Source: CAD feature listing. Evaluate the final solid. Frame: model axes, mm. A direction names the side the tool comes from. Round coordinates to 2 decimals unless told otherwise and drop trailing zeros. Write each loop counter-clockwise with the first axis right and the second up, starting at its lowest first coordinate (ties: lowest second). Pieces come first, ordered by that corner, then holes. Notation, with made-up numbers: M -37,69 L 3,69 A29 cw 3,107 Z; hole C -39,-2 d10. An arc over 180 degrees is marked long. Use a Markdown table: item, result.
```python
from build123d import *

# Parameters (mm, degrees)
SKETCH1_W             = 128
SKETCH1_H             = 2.5
BOSS_EXTRUDE1_DEPTH   = 8
BOSS_EXTRUDE1_2_DEPTH = 8
SKETCH2_W             = 128
SKETCH2_H             = 21
BOSS_EXTRUDE2_DEPTH   = 3
SKETCH3_W             = 21
SKETCH3_H             = 17
BOSS_EXTRUDE3_DEPTH   = 2.5
SKETCH4_W             = 15
SKETCH4_H             = 21
BOSS_EXTRUDE4_DEPTH   = 2.5
SKETCH5_W             = 21
SKETCH5_H             = 39.5
BOSS_EXTRUDE5_DEPTH   = 2.5
FILLET1_R             = 5
SKETCH6_W             = 16
SKETCH6_H             = 8
CUT_EXTRUDE1_DEPTH    = 18.5
FILLET2_R             = 2


with BuildPart() as part:
    # Sketch1 → Boss-Extrude1 (new body)
    with BuildSketch(Plane(origin=(0, 0, 0), x_dir=(1, 0, 0), z_dir=(0, 1, 0))):
        with Locations((10.384615385, 14.211538462)):
            Rectangle(SKETCH1_W, SKETCH1_H)
    extrude(amount=BOSS_EXTRUDE1_DEPTH)



with BuildPart() as body_2:
    # Sketch1 → Boss-Extrude1 2 (new body)
    with BuildSketch(Plane(origin=(0, 0, 0), x_dir=(1, 0, 0), z_dir=(0, 1, 0))):
        with Locations((10.384615385, -4.288461538)):
            Rectangle(SKETCH1_W, SKETCH1_H)
    extrude(amount=BOSS_EXTRUDE1_2_DEPTH)


with BuildPart() as part_1:
    add(part.part)

    add(body_2.part)  # Boss-Extrude2 merges body 2
    # Sketch2 → Boss-Extrude2 (add)
    with BuildSketch(Plane(origin=(0, 8, 0), x_dir=(1, 0, 0), z_dir=(0, 1, 0))):
        with Locations((10.384615385, 4.961538462)):
            Rectangle(SKETCH2_W, SKETCH2_H)
    extrude(amount=BOSS_EXTRUDE2_DEPTH)

    # Sketch3 → Boss-Extrude3 (add)
    with BuildSketch(Plane(origin=(74.384615385, 0, 0), x_dir=(0, 0, -1), z_dir=(1, 0, 0))):
        with Locations((4.961538462, 8.5)):
            Rectangle(SKETCH3_W, SKETCH3_H)
    extrude(amount=BOSS_EXTRUDE3_DEPTH)

    # Sketch4 → Boss-Extrude4 (add)
    with BuildSketch(Plane(origin=(0, 17, 0), x_dir=(1, 0, 0), z_dir=(0, 1, 0))):
        with Locations((69.384615385, 4.961538462)):
            Rectangle(SKETCH4_W, SKETCH4_H)
    extrude(amount=BOSS_EXTRUDE4_DEPTH)

    # Sketch5 → Boss-Extrude5 (add)
    with BuildSketch(Plane(origin=(76.884615385, 0, 0), x_dir=(0, 0, -1), z_dir=(1, 0, 0))):
        with Locations((4.961538462, 9.75)):
            Rectangle(SKETCH5_W, SKETCH5_H)
    extrude(amount=BOSS_EXTRUDE5_DEPTH)

    # Fillet1
    fillet1_edges = [part_1.edges().sort_by_distance(p)[0] for p in [
        (78.134615385, 29.5, 5.538461538),
        (78.134615385, -10, 5.538461538),
        (78.134615385, -10, -15.461538462),
        (78.134615385, 29.5, -15.461538462),
    ]]
    fillet(fillet1_edges, radius=FILLET1_R)

    # Sketch6 → Cut-Extrude1 (cut)
    with BuildSketch(Plane.ZY.offset(-74.384615385)):
        with Locations((-4.961538462, 4)):
            Rectangle(SKETCH6_W, SKETCH6_H)
    extrude(amount=-CUT_EXTRUDE1_DEPTH, mode=Mode.SUBTRACT)

    # Fillet2
    fillet2_edges = [part_1.edges().sort_by_distance(p)[0] for p in [
        (78.134615385, 0, 3.038461538),
        (78.134615385, 0, -12.961538462),
    ]]
    fillet(fillet2_edges, radius=FILLET2_R)


solid = part_1.part
```
Q1. Section B-B on y = 4. Return loops of the section in (x, z), plus the area to 3 significant figures.
Results are:
| item | result |
|---|---|
| outline | M -53.62,-15.46 L 79.38,-15.46 L 79.38,-12.96 L -53.62,-12.96 Z; M -53.62,3.04 L 79.38,3.04 L 79.38,5.54 L -53.62,5.54 Z |
| area | 665 mm^2 |
Q2. Reachability of faces 4 (the flat face through (78, 0, -5)), 5 (the flat face through (74.385, 14, -5)), 6 (the flat face through (18, 6, 5.538)), 7 (the flat face through (11, 0, 4)) from +Z, -Z, +X, -X, +Y, -Y: full face, straight path, thin tool, end or side. Return the list, or none.
Results are:
| item | result |
|---|---|
| face 4 | +X, -X |
| face 5 | +Z, -Z, -X |
| face 6 | +Z, +X, -X, +Y, -Y |
| face 7 | +Z, -Z, -X, -Y |
Q3. Mould query, pull axis Y, two halves, no side actions, for faces 1 (the cylindrical face through (78.15, -8.57, -13.96)), 2 (the flat face through (68, 17, -5)), 3 (the flat face through (76.885, 25, -5)). Classes: +Y half, -Y half, draft (parallel to the pull), parting line (faces both ways), or undercut.
Results are:
| item | result |
|---|---|
| face 1 | -Y half |
| face 2 | undercut |
| face 3 | draft |
Q4. First-contact query: pin 1 Ø0.8 at (x, z) = (20, -14.5) entering from -Y; pin 2 Ø11 at (y, z) = (24.5, -1.5) entering from -X; pin 3 Ø3 at (y, z) = (13.5, -7) entering from -X. Flat tips, straight axial feed; report the tip coordinate or a pass-through.
Results are:
| item | result |
|---|---|
| pin 1 | y = 0 |
| pin 2 | x = 61.88 |
| pin 3 | x = 74.38 |
Q5. Section A-A on x = 68.5. Return loops of the section in (y, z), plus the area to 4 significant figures.
Results are:
| item | result |
|---|---|
| outline | M 0,-15.46 L 11,-15.46 L 11,5.54 L 0,5.54 L 0,3.04 L 8,3.04 L 8,-12.96 L 0,-12.96 Z; M 17,-15.46 L 19.5,-15.46 L 19.5,5.54 L 17,5.54 Z |
| area | 155.5 mm^2 |
Q6. Section C-C on z = -2.5. Return loops of the section in (x, y).
Results are:
| item | result |
|---|---|
| outline | M -53.62,8 L 79.38,8 L 79.38,29.5 L 76.88,29.5 L 76.88,19.5 L 61.88,19.5 L 61.88,17 L 74.38,17 L 74.38,11 L -53.62,11 Z; M 76.88,-10 L 79.38,-10 L 79.38,0 L 76.88,0 Z |
Q7. Line query: L1, parallel to Y at x = 72.5, z = 1.25; L2, parallel to X at y = -0.5, z = -2.25; L3, parallel to Y at x = -36, z = -3. Output: solid intervals per line, ascending.
Results are:
| item | result |
|---|---|
| L1 | 8 to 11, 17 to 19.5 |
| L2 | 76.88 to 79.38 |
| L3 | 8 to 11 |
Q8. Section D-D on x = -33. Return loops of the section in (y, z), plus the area to 3 significant figures.
Results are:
| item | result |
|---|---|
| outline | M 0,-15.46 L 11,-15.46 L 11,5.54 L 0,5.54 L 0,3.04 L 8,3.04 L 8,-12.96 L 0,-12.96 Z |
| area | 103 mm^2 |
